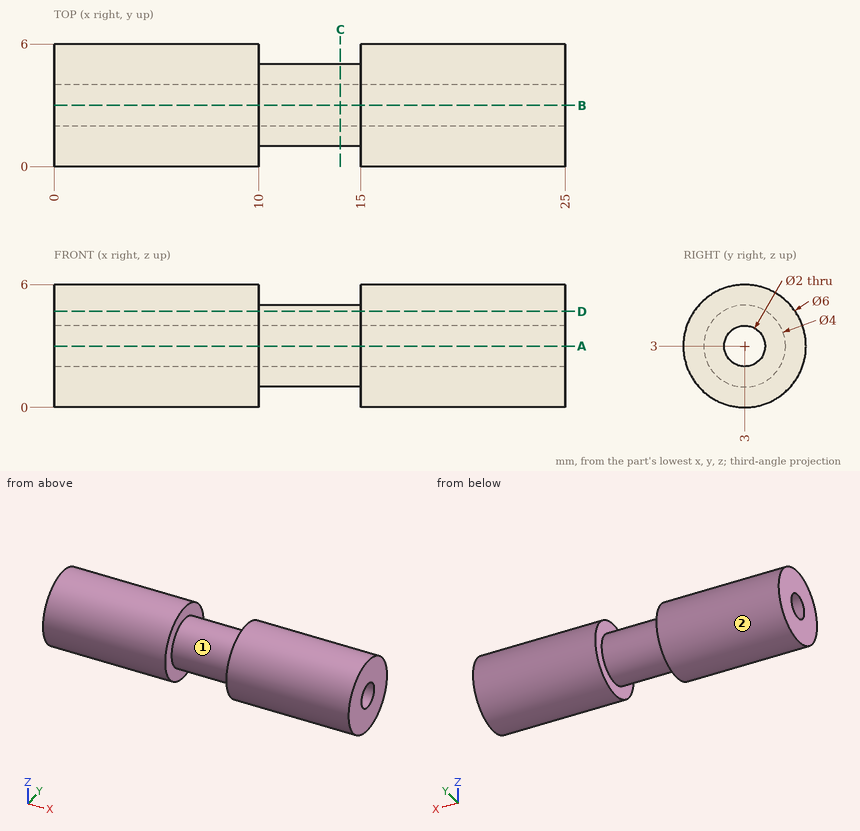
Can you work these out from the drawing? Everything is in mm from the part's minimum corner. A direction names the side the tool comes from. Round coordinates to 2 decimals unless told otherwise and drop trailing zeros. Order: outer loops, then holes, each group sorted by start corner. A loop starts at its lowest first (then second) coordinate and runs counter-clockwise, first axis right, second up. Notation, with made-up numbers: (24, 43.5) - (72, 43.5) arc R29 ccw to (72, 79.5) - close; hole circle Ø5 at (66, 64). An arc over 180 degrees is marked (long way). Answer in a Markdown table with one row per item.
(1) Please list where these lines run through material, in increasing order: L1, parallel to X at y = 5.25, z = 3.95; L2, parallel to Z at x = 5.5, y = 3; L3, parallel to Z at x = 12.5, y = 3. Write a range as from..to.
From the geometry:
| item | result |
|---|---|
| L1 | x = 0..10, 15..25 |
| L2 | z = 0..2, 4..6 |
| L3 | z = 1..2, 4..5 |
(2) Suppose I cut it at A-A, the plane z = 3. Please give me the cut outline in (x, y).
From the geometry:
| item | result |
|---|---|
| outline | (0, 0) - (10, 0) - (10, 1) - (15, 1) - (15, 0) - (25, 0) - (25, 2) - (0, 2) - close; (0, 4) - (25, 4) - (25, 6) - (15, 6) - (15, 5) - (10, 5) - (10, 6) - (0, 6) - close |
(3) Suppose I cut it at C-C, the plane x = 14. Please give me the cut outline in (y, z).
From the geometry:
| item | result |
|---|---|
| outline | circle Ø4 at (3, 3); hole circle Ø2 at (3, 3) |
(4) Suppose I cut it at D-D, the plane z = 4.7. Please give me the cut outline in (x, y), plus the area to 3 significant figures.
From the geometry:
| item | result |
|---|---|
| outline | (0, 0.53) - (10, 0.53) - (10, 1.95) - (15, 1.95) - (15, 0.53) - (25, 0.53) - (25, 5.47) - (15, 5.47) - (15, 4.05) - (10, 4.05) - (10, 5.47) - (0, 5.47) - close |
| area | 109 mm2 |
(5) Which directions (+Z, -Z, +X, -X, +Y, -Y) give clear straight access to the entire face, cutting with the end or side of a thin tool? Please do the marked faces 1 and 2.
From the geometry:
| item | result |
|---|---|
| face 1 | none |
| face 2 | +X, -X |
(6) For P1, Ø3, axis at x = 3, z = 0.5, coming from the -Y side, with a flat end and sliding along its axis, tell me the tip position at first contact or that it passes through.
From the geometry:
| item | result |
|---|---|
| P1 | stops at y = 0.17 |
